Design review of the part built by this model. Coordinates are the model's own, in mm. A direction names the side the tool comes from. Coordinates: 2 decimals unless noted, no trailing zeros. Loops run counter-clockwise (first coordinate to the right, second up) from the corner with the lowest first, then second, coordinate; pieces in that order, holes last. Notation, with made-up numbers: (-34, -1) - (5, -1) arc R12 ccw to (5, 6) - close; hole circle Ø11 at (17, -13.5). An arc over 180 degrees is marked (long way). Answer in a Markdown table with one row per item. Add a question column.
(1) The part is to be moulded in two halves that separate along Z. For faces 1 (the face through (12.325, 0.741, 14.818)), 2 (the face through (5.1, 80.7, 14.8)), 3 (the face through (6.5, 0.8, 3.1)), say which applies: released by +Z, released by -Z, zero draft, split by the parting line, or undercut.
(2) We need section D-D, the plane z = -8.5. Write out the cut boundary in (x, y).
(3) We need section A-A, the plane x = 6.5. Write out the cut boundary in (y, z).
(4) We need section B-B, the plane z = -3. Write out the cut boundary in (x, y), plus the area to 3 significant figures.
(5) We need section C-C, the plane x = 18.5. Write out the cut boundary in (y, z).
(6) For faces 4 (the face through (1, 1, -13)), 5 (the face through (24, 1, -13)), 6 (the face through (12, 50, 14)), 7 (the face through (15, 85.6, 15)), 8 (the face through (6.5, 0.8, -6.1)), list the 3-axis set-ups (+Z, -Z, +X, -X, +Y, -Y) from which the entire face can be reached by the end or side of a thin tool; tool diameter is ignored.
(7) To check wall thickness, follow L1, parallel to Y at x = 3, z = -10.75; L2, parallel to Z at x = 19.75, y = 42.5. State the ranges of each line that lie inside material, in increasing order. Write a range as [from, to].
(8) Clearance check with flat-ended pins moving along their axes: pin 1 (5 mm diameter, centred on x = 21.5, z = -6.5, fed in from -Y); pin 2 (8 mm diameter, centred on x = 22.5, z = -6, fed in from +Y); pin 3 (8 mm diameter, centred on x = 6.5, y = 41, fed in from -Z); pin 4 (0.5 mm diameter, centred on y = 90, z = 15, fed in from -X). State where each tip first meets the part, or that it passes through.
from build123d import *

# Parameters (mm, degrees)
SKETCH_1_W                       = 25
SKETCH_1_H                       = 1.6
SM_BASE_FLANGE_1_DEPTH           = 14
CUT_EXTRUDE_2_REACH              = 30.698
SM_EDGE_FLANGE_1_STRIP_W         = 8.4
SM_EDGE_FLANGE_1_STRIP_H         = 1.6
SM_EDGE_FLANGE_1_STRIP_CUT_DEPTH = 25
SM_EDGE_FLANGE_1_DEPTH           = 25
CUT_EXTRUDE_1_REACH              = 104.705
SKETCH_10_W                      = 20
SKETCH_10_H                      = 10
CHAMFER_1_SIZE                   = 10
CHAMFER_2_SIZE                   = 2


# Sheet-metal steps are written as plain solids
with BuildPart() as part:
    # Sketch 1 → 基材-凸緣1 (new, symmetric)
    with BuildSketch(Plane.XY):
        with Locations((12.5, 0.8)):
            Rectangle(SKETCH_1_W, SKETCH_1_H)
    extrude(amount=SM_BASE_FLANGE_1_DEPTH, both=True)

    # 草圖11 → 除料-伸長2 (cut, up to next)
    with BuildSketch(Plane.XZ, mode=Mode.PRIVATE) as cut_extrude_2_sk1:
        with BuildLine():
            Line((16.4, 1), (16.4, -4))
            ThreePointArc((16.4, -4), (18.5, -6.1), (20.6, -4))
            Line((20.6, -4), (20.6, 1))
            ThreePointArc((20.6, 1), (18.5, 3.1), (16.4, 1))
        make_face()
    cut_extrude_2_tool1 = extrude(cut_extrude_2_sk1.sketch, amount=-CUT_EXTRUDE_2_REACH, mode=Mode.PRIVATE) & part.part
    # 草圖11 → 除料-伸長2 (cut, up to next)
    with BuildSketch(Plane.XZ, mode=Mode.PRIVATE) as cut_extrude_2_sk2:
        with BuildLine():
            Line((4.4, 1), (4.4, -4))
            ThreePointArc((4.4, -4), (6.5, -6.1), (8.6, -4))
            Line((8.6, -4), (8.6, 1))
            ThreePointArc((8.6, 1), (6.5, 3.1), (4.4, 1))
        make_face()
    cut_extrude_2_tool2 = extrude(cut_extrude_2_sk2.sketch, amount=-CUT_EXTRUDE_2_REACH, mode=Mode.PRIVATE) & part.part
    add(cut_extrude_2_tool1.solids().sort_by_distance((18.5, 0, -1.5))[0], mode=Mode.SUBTRACT)
    add(cut_extrude_2_tool2.solids().sort_by_distance((6.5, 0, -1.5))[0], mode=Mode.SUBTRACT)

    # 邊線-凸緣1 strip (across the edge) → 邊線-凸緣1 strip cut (cut)
    with BuildSketch(Plane(origin=(0, 1.6, 14), x_dir=(0, 0, -1), z_dir=(1, 0, 0))):
        with Locations((-3.2, -0.8)):
            Rectangle(SM_EDGE_FLANGE_1_STRIP_W, SM_EDGE_FLANGE_1_STRIP_H)
    extrude(amount=SM_EDGE_FLANGE_1_STRIP_CUT_DEPTH, mode=Mode.SUBTRACT)

    # 邊線-凸緣1 section (across the edge) → 邊線-凸緣1 (add)
    with BuildSketch(Plane(origin=(0, 1.6, 14), x_dir=(0, 0, -1), z_dir=(1, 0, 0))):
        with BuildLine():
            Line((-1.6, 1), (-1.6, 94))
            Line((-1.6, 94), (0, 94))
            Line((0, 94), (0, 1))
            ThreePointArc((0, 1), (0.292893219, 0.292893219), (1, 0))
            Line((1, 0), (1, -1.6))
            ThreePointArc((1, -1.6), (-0.838477631, -0.838477631), (-1.6, 1))
        make_face()
    extrude(amount=SM_EDGE_FLANGE_1_DEPTH)

    # 草圖10 → 除料-伸長1 (cut, up to next)
    with BuildSketch(Plane(origin=(0, 0, 14), x_dir=(-1, 0, 0), z_dir=(0, 0, -1)), mode=Mode.PRIVATE) as cut_extrude_1_sk1:
        with Locations((-10, 90.6)):
            Rectangle(SKETCH_10_W, SKETCH_10_H)
    cut_extrude_1_tool1 = extrude(cut_extrude_1_sk1.sketch, amount=-CUT_EXTRUDE_1_REACH, mode=Mode.PRIVATE) & part.part
    add(cut_extrude_1_tool1.solids().sort_by_distance((10, 90.6, 14))[0], mode=Mode.SUBTRACT)

    # 導角1
    chamfer_1_edges = [part.edges().sort_by_distance(p)[0] for p in [
        (0, 85.6, 14.8),
    ]]
    chamfer(chamfer_1_edges, length=CHAMFER_1_SIZE)

    # 導角2
    chamfer_2_edges = [part.edges().sort_by_distance(p)[0] for p in [
        (25, 0.8, -14),
        (0, 0.8, -14),
    ]]
    chamfer(chamfer_2_edges, length=CHAMFER_2_SIZE)


solid = part.part
Responses:
| question | item | result |
|---|---|---|
| 1 | face 1 | released by +Z |
| 1 | face 2 | zero draft |
| 1 | face 3 | undercut |
| 2 | outline | (0, 0) - (25, 0) - (25, 1.6) - (0, 1.6) - close |
| 3 | outline | (0, -14) - (1.6, -14) - (1.6, -6.1) - (0, -6.1) - close; (0, 3.1) - (1.6, 3.1) - (1.6, 13) arc R1 cw to (2.6, 14) - (82.1, 14) - (82.1, 15.6) - (2.6, 15.6) arc R2.6 ccw to (0, 13) - close |
| 4 | outline | (0, 0) - (4.4, 0) - (4.4, 1.6) - (0, 1.6) - close; (8.6, 0) - (16.4, 0) - (16.4, 1.6) - (8.6, 1.6) - close; (20.6, 0) - (25, 0) - (25, 1.6) - (20.6, 1.6) - close |
| 4 | area | 26.6 mm2 |
| 5 | outline | (0, -14) - (1.6, -14) - (1.6, -6.1) - (0, -6.1) - close; (0, 3.1) - (1.6, 3.1) - (1.6, 13) arc R1 cw to (2.6, 14) - (85.6, 14) - (85.6, 15.6) - (2.6, 15.6) arc R2.6 ccw to (0, 13) - close |
| 6 | face 4 | -Z, -X, +Y, -Y |
| 6 | face 5 | -Z, +X, +Y, -Y |
| 6 | face 6 | -Z, +X, -X, +Y |
| 6 | face 7 | +Z, -Z, -X, +Y |
| 6 | face 8 | +Y, -Y |
| 7 | L1 | y = [0, 1.6] |
| 7 | L2 | z = [14, 15.6] |
| 8 | pin 1 | stops at y = 0 |
| 8 | pin 2 | stops at y = 1.6 |
| 8 | pin 3 | stops at z = 14 |
| 8 | pin 4 | stops at x = 20 |
